Geometry check sheet. Reference: drawing and pictorial views, mm from the part's lowest x, y, z. A direction names the side the tool comes from. Round coordinates to 2 decimals unless told otherwise and drop trailing zeros. Order: outer loops, then holes, each group sorted by start corner. A loop starts at its lowest first (then second) coordinate and runs counter-clockwise, first axis right, second up.
(1) Set-up check for the marked faces 5, 6, 7 and 8: record each of +Z, -Z, +X, -X, +Y, -Y from which the full face is reachable in a straight line by a thin tool's end or side.
(2) Gauge pin test, flat ends, axial feed: P1, Ø2.5, axis at y = 7.5, z = 12.5, coming from the +X side; P2, Ø2.5, axis at y = 73.5, z = 45, coming from the +X side; P3, Ø1.5, axis at y = 60.5, z = 10, coming from the +X side. Record the tip position at first contact, or that the pin passes through.
(3) Cross-section at A-A on x = 28. Enter the section's corners in (y, z).
(4) Draft check along X on the marked faces 1, 2, 3 and 4. Enter one of: pulls with the +X half, pulls with the -X half, needs draft (parallel to the pull), parting line crosses it, or undercut.
(5) Thickness scan on L1, parallel to Y at x = 29.5, z = 7; L2, parallel to Z at x = 26.5, y = 75.5; L3, parallel to Z at x = 15, y = 67.5. Record the ranges inside material, lowest first.
(6) Cross-section at D-D on x = 12. Enter the section's corners in (y, z).
(7) Cross-section at C-C on z = 11. Enter the section's corners in (x, y), and give its area (3 significant figures).
(8) Cross-section at B-B on y = 63. Enter the section's corners in (x, z).
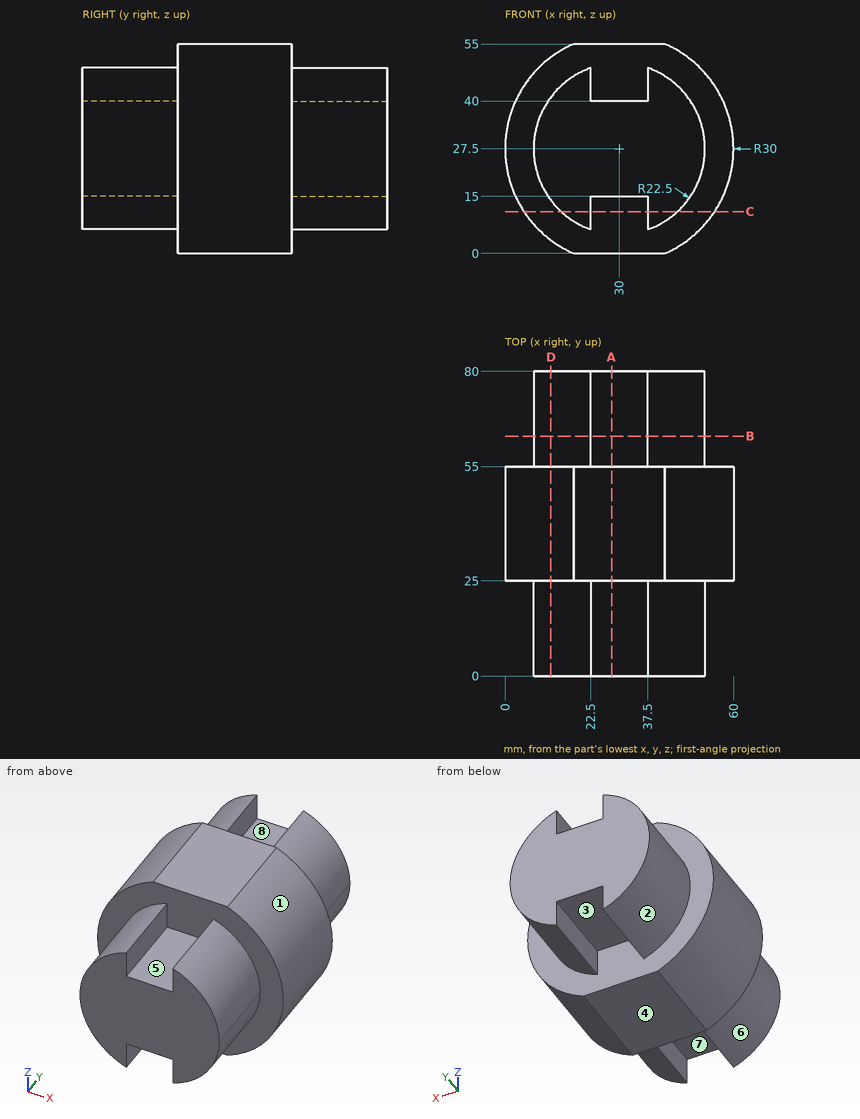
Found:
1. face 5: +Z, -Y
1. face 6: -X, -Y
1. face 7: -Z, -Y
1. face 8: +Z, +Y
2. P1: stops at x = 47.81
2. P2: stops at x = 45.56
2. P3: stops at x = 45.02
3. outline: (0, 15) - (25, 15) - (25, 0) - (55, 0) - (55, 15) - (80, 15) - (80, 40) - (55, 40) - (55, 55) - (25, 55) - (25, 40) - (0, 40) - close
4. face 1: pulls with the +X half
4. face 2: pulls with the -X half
4. face 3: undercut
4. face 4: needs draft
5. L1: y = 25 to 55
5. L2: z = 15 to 40
5. L3: z = 10.73 to 44.27
6. outline: (0, 14) - (25, 14) - (25, 3.5) - (55, 3.5) - (55, 14) - (80, 14) - (80, 41) - (55, 41) - (55, 51.5) - (25, 51.5) - (25, 41) - (0, 41) - close
7. outline: (4.95, 25) - (14.7, 25) - (14.7, 0) - (22.5, 0) - (22.5, 25) - (37.5, 25) - (37.5, 0) - (45.3, 0) - (45.3, 25) - (55.05, 25) - (55.05, 55) - (45.3, 55) - (45.3, 80) - (37.5, 80) - (37.5, 55) - (22.5, 55) - (22.5, 80) - (14.7, 80) - (14.7, 55) - (4.95, 55) - close
7. area: 2,280 mm2
8. outline: (22.5, 6.29) - (22.5, 15) - (37.5, 15) - (37.5, 6.29) arc R22.5 ccw to (37.5, 48.71) - (37.5, 40) - (22.5, 40) - (22.5, 48.71) arc R22.5 ccw to start
